Source: CAD feature listing. Evaluate the final solid. Frame: model axes, mm. Face numbers are marked on the shaded views. A direction names the side the tool comes from. Round coordinates to 2 decimals unless told otherwise and drop trailing zeros. Write each loop counter-clockwise with the first axis right and the second up, starting at its lowest first coordinate (ties: lowest second). Pieces come first, ordered by that corner, then holes. Notation, with made-up numbers: M 58,77 L 97,77 A26 ccw 97,91 Z; hole C -22.75,-13.75 d10. An arc over 180 degrees is marked long. Answer in a Markdown table with one row per item. Add a question column.
Item 1: Cut plane A-A on z = 1. Return loops of the section in (x, y).
Item 2: Cut plane C-C on x = -3.5. Return loops of the section in (y, z), and give its area (3 significant figures).
Item 3: Mould query, pull axis Y, two halves, no side actions, for the marked faces 6, 7 and 8. Classes: released by +Y, released by -Y, zero draft, split by the parting line, or undercut.
Item 4: Cut plane B-B on y = 0. Return loops of the section in (x, z), and give its area (3 significant figures).
Item 5: Set-up query: the marked faces 1, 2, 3, 4 and 5. Return all of +Z, -Z, +X, -X, +Y, -Y with unobstructed straight access to the full face (end or side cutting, diameter ignored); none if empty.
Item 6: Cut plane D-D on z = 8. Return loops of the section in (x, y), and give its area (3 significant figures).
Item 7: Contact query for flat-ended pins moving along their axis: pin 1 (1.6 mm diameter, centred on x = -4.5, z = 1.5, fed in from -Y); pin 2 (3 mm diameter, centred on x = 3, y = 7, fed in from +Z); pin 3 (3 mm diameter, centred on x = 0.5, y = -1, fed in from -Z). Output: stop coordinate, or through.
Item 8: Material intervals for probe 1 along X at (y, z) = (0, 8.75); probe 2 along Z at (x, y) = (-1.5, -2); probe 3 along Y at (x, z) = (-2.5, 1.25), sorted ascending.
from build123d import *

# Parameters (mm, degrees)
PAD005_DEPTH    = 10
POCKET002_DEPTH = 4
SKETCH010_R     = 1.65
POCKET003_DEPTH = 6.201


with BuildPart() as part:
    # Sketch008 → Pad005 (new body, symmetric)
    with BuildSketch(Plane.YZ):
        Polygon((-6.5, 0), (-6.5, 2), (-9.5, 3.7), (-9.5, 6.2), (-4, 6.2), (-4, 10.2), (0, 10.2), (0, 0), align=None)
    pad005 = extrude(amount=PAD005_DEPTH, both=True)

    # Mirrored: Pad005 across Sketch008 V_Axis
    add(pad005.mirror(Plane(origin=(0, 0, 0), x_dir=(1, 0, 0), z_dir=(0, 1, 0))))

    # Sketch009 (on Face2 of Mirrored) → Pocket002 (cut)
    with BuildSketch(Plane.YX):
        Polygon((-1.732051, 3), (-3.464102, 0), (-1.732051, -3), (1.732051, -3), (3.464102, 0), (1.732051, 3), align=None)
    extrude(amount=-POCKET002_DEPTH, mode=Mode.SUBTRACT)

    # Sketch010 (on Face20 of Pocket002) → Pocket003 (cut, through all)
    with BuildSketch(Plane.YX.offset(-4)):
        Circle(SKETCH010_R)
    extrude(amount=-POCKET003_DEPTH, mode=Mode.SUBTRACT)


solid = part.part
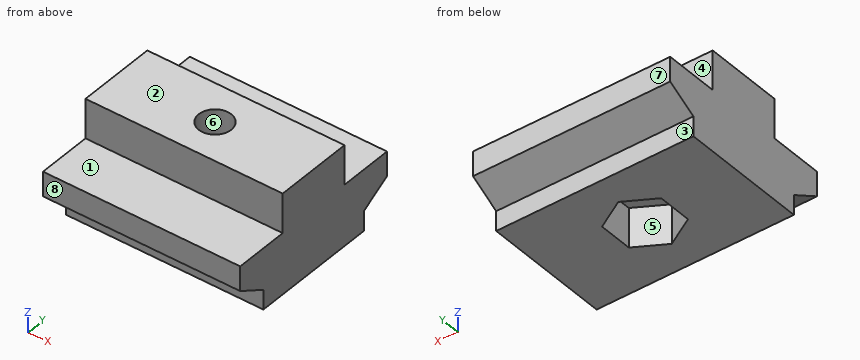
Results below:
| question | item | result |
|---|---|---|
| 1 | outline | M -10,-6.5 L 10,-6.5 L 10,6.5 L -10,6.5 Z; hole M -3,-1.73 L 0,-3.46 L 3,-1.73 L 3,1.73 L 0,3.46 L -3,1.73 Z |
| 2 | outline | M -9.5,3.7 L -6.5,2 L -6.5,0 L 6.5,0 L 6.5,2 L 9.5,3.7 L 9.5,6.2 L 4,6.2 L 4,10.2 L -4,10.2 L -4,6.2 L -9.5,6.2 Z |
| 2 | area | 133 mm2 |
| 3 | face 6 | undercut |
| 3 | face 7 | released by +Y |
| 3 | face 8 | released by -Y |
| 4 | outline | M -10,0 L -3,0 L -3,4 L -1.65,4 L -1.65,10.2 L -10,10.2 Z; M 1.65,4 L 3,4 L 3,0 L 10,0 L 10,10.2 L 1.65,10.2 Z |
| 4 | area | 160 mm2 |
| 5 | face 1 | +Z, +X, -X, -Y |
| 5 | face 2 | +Z, +X, -X, +Y, -Y |
| 5 | face 3 | -Z, +X, -X, +Y |
| 5 | face 4 | +Z, +X, -X, +Y |
| 5 | face 5 | -Z |
| 6 | outline | M -10,-4 L 10,-4 L 10,4 L -10,4 Z; hole C 0,0 d3.3 |
| 6 | area | 151 mm2 |
| 7 | pin 1 | y = -7.03 |
| 7 | pin 2 | z = 6.2 |
| 7 | pin 3 | z = 4 |
| 8 | probe 1 | -10 to -1.65, 1.65 to 10 |
| 8 | probe 2 | 4 to 10.2 |
| 8 | probe 3 | -6.5 to -2.02, 2.02 to 6.5 |
